from build123d import *

# Parameters (mm, degrees)
F1_DEPTH = 247.65
F2_R     = 63.5
F2_W     = 254
F2_H     = 127
F3_DEPTH = 48.261
F4_R     = 38.1
F5_DEPTH = 218.44
F6_R     = 127


with BuildPart() as f1:
    # F0 (on Front) → F1 (new body, symmetric)
    with BuildSketch(Plane.XZ):
        with BuildLine():
            ThreePointArc((-85.393344, 183.85906), (-101.36096, 64.6829), (0, 0))
            Line((0, 0), (1270, 0))
            Line((1270, 0), (1270, 48.26))
            Line((1270, 48.26), (6.174015, 48.26))
            ThreePointArc((6.174015, 48.26), (-55.52241, 80.333411), (-51.264285, 149.738173))
            Line((-51.264285, 149.738173), (397.744435, 598.746893))
            Line((397.744435, 598.746893), (363.619462, 632.871866))
            Line((363.619462, 632.871866), (-85.393344, 183.85906))
        make_face()
    extrude(amount=F1_DEPTH, both=True)

    # F2 (on face) → F3 (cut, through all)
    with BuildSketch(Plane.XY.offset(48.26)):
        with Locations((457.2, 0)):
            Circle(F2_R)
        with Locations((974.09, 0)):
            Rectangle(F2_W, F2_H)
        with BuildLine():
            Line((847.09, -63.5), (847.09, 63.5))
            ThreePointArc((847.09, 63.5), (783.59, 0), (847.09, -63.5))
        make_face()
        with BuildLine():
            ThreePointArc((1101.09, -63.5), (1164.59, 0), (1101.09, 63.5))
            Line((1101.09, 63.5), (1101.09, -63.5))
        make_face()
    extrude(amount=-F3_DEPTH, mode=Mode.SUBTRACT)

    # F4 (on face) → F5 (cut)
    with BuildSketch(Plane(origin=(-134.626202, 0, 134.626202), x_dir=(0, -1, 0), z_dir=(-0.707107, 0, 0.707107))):
        with Locations((-133.35, 514.125775)):
            Circle(F4_R)
        with Locations((133.35, 514.125775)):
            Circle(F4_R)
    extrude(amount=-F5_DEPTH, mode=Mode.SUBTRACT)

    # F6
    f6_edges = [f1.edges().sort_by_distance(p)[0] for p in [
        (380.681949, -247.65, 615.809379),
        (380.681949, 247.65, 615.809379),
        (1270, 247.65, 24.13),
        (1270, -247.65, 24.13),
    ]]
    fillet(f6_edges, radius=F6_R)


solid = f1.part
Source: CAD feature listing. Evaluate the final solid. Frame: model axes, mm. A direction names the side the tool comes from. Coordinates: 2 decimals unless noted, no trailing zeros. Loops run counter-clockwise (first coordinate to the right, second up) from the corner with the lowest first, then second, coordinate; pieces in that order, holes last. Notation, with made-up numbers: (58.5, 25.25) -> (111.5, 25.25) arc R13 cw to (111.5, 41.25) -> close; hole circle Ø10 at (54.25, 13.25). An arc over 180 degrees is marked (long way). Answer in a Markdown table with one row per item. Add a question column.
Q1. Ray query, line 1 along Y through (x, z) = (457, 20); line 2 along Z through (x, y) = (1012.5, 90.5). Return the intervals inside material, ascending.
Q2. Contact query for flat-ended pins moving along their axis: pin 1 Ø8 at (y, z) = (90, 440) entering from -X; pin 2 Ø4 at (y, z) = (-74.5, 146) entering from +X; pin 3 Ø8 at (y, z) = (112.5, 281.5) entering from +X. Output: stop coordinate, or through.
Q3. Section A-A on y = 0. Return the cut outline in (x, z), and give its area (3 significant figures).
Q4. Section B-B on x = 457.2. Return the cut outline in (y, z), and give its area (3 significant figures).
Q5. Section D-D on y = 197.5. Return the cut outline in (x, z), and give its area (3 significant figures).
Q6. Reachability of faces 4 (the face through (972, -63.5, 24)), 5 (the face through (647, -3, 48.26)), 6 (the face through (626, -3, 0)) from +Z, -Z, +X, -X, +Y, -Y: full face, straight path, thin tool, end or side. Return the list, or none.
Q7. Pull-direction query (Y, two-part tool) for faces 1 (the face through (1231.81, -211.435, 24.468)), 2 (the face through (353.438, 211.435, 589.044)), 3 (the face through (972, 63.5, 24)); classes: pulls with the +Y half, pulls with the -Y half, needs draft (parallel to the pull), parting line crosses it, or undercut.
Q8. Section C-C on z = 207. Return the cut outline in (x, y), and give its area (3 significant figures).
Computed values:
| question | item | result |
|---|---|---|
| 1 | line 1 | y = -247.65 to -63.5, 63.5 to 247.65 |
| 1 | line 2 | z = 0 to 48.26 |
| 2 | pin 1 | stops at x = 166.75 |
| 2 | pin 2 | stops at x = -52.51 |
| 2 | pin 3 | stops at x = 84.5 |
| 3 | outline | (-85.39, 183.86) arc R111.76 ccw to (0, 0) -> (393.7, 0) -> (393.7, 48.26) -> (6.17, 48.26) arc R63.8 cw to (-51.26, 149.74) -> (397.74, 598.75) -> (363.62, 632.87) -> close; (520.7, 0) -> (783.59, 0) -> (783.59, 48.26) -> (520.7, 48.26) -> close; (1164.59, 0) -> (1270, 0) -> (1270, 48.26) -> (1164.59, 48.26) -> close |
| 3 | area | 76,900 mm^2 |
| 4 | outline | (-247.65, 0) -> (-63.5, 0) -> (-63.5, 48.26) -> (-247.65, 48.26) -> close; (63.5, 0) -> (247.65, 0) -> (247.65, 48.26) -> (63.5, 48.26) -> close |
| 4 | area | 17,800 mm^2 |
| 5 | outline | (-85.39, 183.86) arc R111.76 ccw to (0, 0) -> (1244.11, 0) -> (1244.11, 48.26) -> (6.17, 48.26) arc R63.8 cw to (-51.26, 149.74) -> (379.44, 580.44) -> (345.31, 614.56) -> close |
| 5 | area | 98,900 mm^2 |
| 6 | face 4 | +Z, -Z |
| 6 | face 5 | +X, +Y, -Y |
| 6 | face 6 | -Z, +X, -X, +Y, -Y |
| 7 | face 1 | pulls with the -Y half |
| 7 | face 2 | pulls with the +Y half |
| 7 | face 3 | undercut |
| 8 | outline | (-62.25, -247.65) -> (6, -247.65) -> (6, 247.65) -> (-62.25, 247.65) -> close |
| 8 | area | 33,800 mm^2 |
